Work out the finished part from the listing and answer in its coordinate system (mm). A direction names the side the tool comes from. Give positions to 0.01 mm unless a question says otherwise; leave off trailing zeros. Loops run counter-clockwise (first coordinate to the right, second up) from the corner with the lowest first, then second, coordinate; pieces in that order, holes last. Notation, with made-up numbers: (6, 18.5) - (41, 18.5) arc R22 ccw to (41, 50.5) - close; hole circle Ø7 at (2.25, 25.25). An arc over 180 degrees is marked (long way). One line per item, written item: value.
from build123d import *

# Parameters (mm, degrees)
SKETCH_R           = 98.425
PAD_DEPTH          = 0.6
PAD001_DEPTH       = 5
POLARPATTERN_COUNT = 4
SKETCH002_R        = 28
POCKET_DEPTH       = 5.601
SKETCH003_W        = 15
SKETCH003_H        = 24
POCKET001_DEPTH    = 5.601
POCKET002_DEPTH    = 5
POCKET003_DEPTH    = 5


with BuildPart() as part:
    # Sketch → Pad (new body)
    with BuildSketch(Plane.XY):
        Circle(SKETCH_R)
    extrude(amount=-PAD_DEPTH)

    # Sketch001 → Pad001 (new body)
    with BuildSketch(Plane.XY):
        with BuildLine():
            ThreePointArc((3.175, -21.997045), (15.715448, -15.715448), (21.997045, -3.175))
            Line((21.997045, -3.175), (98.373777, -3.175))
            ThreePointArc((3.175, -98.373777), (69.596985, -69.596985), (98.373777, -3.175))
            Line((3.175, -21.997045), (3.175, -98.373777))
        make_face()
    pad001 = extrude(amount=PAD001_DEPTH)

    # PolarPattern: Pad001 ×4 about axis
    polarpattern_axis = Axis((0, 0, 0), (0, 0, 1))
    for i in range(1, POLARPATTERN_COUNT):
        add(pad001.rotate(polarpattern_axis, i * 360 / POLARPATTERN_COUNT))

    # Sketch002 → Pocket (cut, through all)
    with BuildSketch(Plane.XY.offset(5)):
        Circle(SKETCH002_R)
    extrude(amount=-POCKET_DEPTH, mode=Mode.SUBTRACT)

    # Sketch003 → Pocket001 (cut, through all)
    with BuildSketch(Plane(origin=(0, 0, -0.6), x_dir=(1, 0, 0), z_dir=(0, 0, -1))):
        with Locations((97.5, 0)):
            Rectangle(SKETCH003_W, SKETCH003_H)
    extrude(amount=-POCKET001_DEPTH, mode=Mode.SUBTRACT)

    # Sketch004 → Pocket002 (cut)
    with BuildSketch(Plane.XY.offset(5)):
        with BuildLine():
            ThreePointArc((8.175, -31.971384), (15.237308, -29.271564), (21.499759, -25.035183))
            Line((21.499759, -25.035183), (64.270084, -67.805508))
            ThreePointArc((8.175, -93.066643), (38.361488, -85.185837), (64.270084, -67.805508))
            Line((8.175, -31.971384), (8.175, -93.066643))
        make_face()
        with BuildLine():
            ThreePointArc((25.035284, -21.499641), (29.2716, -15.237239), (31.971384, -8.175))
            Line((31.971384, -8.175), (85, -8.175))
            Line((85, -17), (85, -8.175))
            Line((85, -17), (91.865285, -17))
            ThreePointArc((67.805615, -64.269971), (83.260505, -42.378284), (91.865285, -17))
            Line((25.035284, -21.499641), (67.805615, -64.269971))
        make_face()
    pocket002 = extrude(amount=-POCKET002_DEPTH, mode=Mode.SUBTRACT)

    # Mirrored: Pocket002 across Sketch004 H_Axis
    add(pocket002.mirror(Plane(origin=(0, 0, 5), x_dir=(0, 0, 1), z_dir=(0, 1, 0))), mode=Mode.SUBTRACT)

    # Sketch005 → Pocket003 (cut)
    with BuildSketch(Plane.XY.offset(5)):
        with BuildLine():
            ThreePointArc((-31.971384, -8.175), (-29.271564, -15.237308), (-25.035182, -21.49976))
            Line((-25.035182, -21.49976), (-67.805507, -64.270085))
            ThreePointArc((-93.066643, -8.175), (-85.185837, -38.361489), (-67.805507, -64.270085))
            Line((-93.066643, -8.175), (-31.971384, -8.175))
        make_face()
        with BuildLine():
            ThreePointArc((-21.49964, -25.035285), (-15.237238, -29.2716), (-8.175, -31.971384))
            Line((-8.175, -31.971384), (-8.175, -93.066643))
            ThreePointArc((-64.26997, -67.805616), (-38.361417, -85.185869), (-8.175, -93.066643))
            Line((-21.49964, -25.035285), (-64.26997, -67.805616))
        make_face()
    pocket003 = extrude(amount=-POCKET003_DEPTH, mode=Mode.SUBTRACT)

    # Mirrored001: Pocket003 across Sketch005 H_Axis
    add(pocket003.mirror(Plane(origin=(0, 0, 5), x_dir=(0, 0, 1), z_dir=(0, 1, 0))), mode=Mode.SUBTRACT)


solid = part.part
1. For faces 3 (the flat face through (-63, -3.175, 2)), 4 (the flat face through (-3.175, 63, 2)), 5 (the cylindrical face through (29.222, -15.331, 2.535)), determine the directions among +Z, -Z, +X, -X, +Y, -Y from which every point of the face is accessible in a straight line to the end or side of a thin tool.
Output:
face 3: +Z, +X, -X
face 4: +Z, +Y, -Y
face 5: +Z
2. The mould has two halves that part along Y. Classify faces 1 (the flat face through (46.121, -42.585, 2.535)), 2 (the flat face through (-47, 47, 5)): released by +Y, released by -Y, zero draft, split by the parting line, or undercut.
Output:
face 1: undercut
face 2: zero draft
3. Flat-ended cylindrical pins translate along their axes: pin 1 Ø1.9 at (x, y) = (-1, 51) entering from +Z; pin 2 Ø2 at (y, z) = (-25, 1) entering from +X; pin 3 Ø1.5 at (y, z) = (58, 3) entering from -X; pin 4 Ø17 at (x, y) = (-48, 33.5) entering from +Z. Find the tip coordinate at first contact, or state that the pin passes through.
Output:
pin 1: stops at z = 0
pin 2: stops at x = 95.45
pin 3: stops at x = -80.06
pin 4: stops at z = 5
4. Section D-D (x = 46) is taken. Write down the section's boundary in (y, z) (3 decimals).
Output:
outline: (-87.014, -0.6) - (87.014, -0.6) - (87.014, 5) - (81.316, 5) - (81.316, 0) - (49.535, 0) - (49.535, 5) - (42.464, 5) - (42.464, 0) - (8.175, 0) - (8.175, 5) - (3.175, 5) - (3.175, 0) - (-3.175, 0) - (-3.175, 5) - (-8.175, 5) - (-8.175, 0) - (-42.464, 0) - (-42.464, 5) - (-49.535, 5) - (-49.535, 0) - (-81.316, 0) - (-81.316, 5) - (-87.014, 5) - close
5. Section B-B (x = 0) is taken. Write down the section's boundary in (y, z) (3 decimals).
Output:
outline: (-98.425, -0.6) - (-28, -0.6) - (-28, 0) - (-98.425, 0) - close; (28, -0.6) - (98.425, -0.6) - (98.425, 0) - (28, 0) - close
6. Section C-C (z = 2.3) is taken. Count the separate pieces of the cut face and the enclosed holes in it, and give its area (3 significant figures).
Output:
separate pieces: 4
enclosed holes: 8
area: 7,350 mm²
7. Find the intervals of material crossed by line 1 along X through (y, z) = (22.5, 2.3); line 2 along Y through (x, z) = (-45.5, 3.6) (3 decimals); line 3 along Y through (x, z) = (30, 0.5) (3 decimals), in increasing order.
Output:
line 1: x = -95.82 to -90.68, -26.04 to -16.67, 16.67 to 26.04, 90.68 to 95.82
line 2: y = -87.277 to -81.596, -49.036 to -41.965, -8.175 to -3.175, 3.175 to 8.175, 41.965 to 49.036, 81.596 to 87.277
line 3: y = -93.742 to -88.477, -33.535 to -26.464, -13.748 to -3.175, 3.175 to 13.748, 26.464 to 33.535, 88.477 to 93.742
8. Section A-A (y = 0) is taken. Write down the section's boundary in (x, z) (3 decimals).
Output:
outline: (-98.425, -0.6) - (-28, -0.6) - (-28, 0) - (-98.425, 0) - close; (28, -0.6) - (90, -0.6) - (90, 0) - (28, 0) - close
